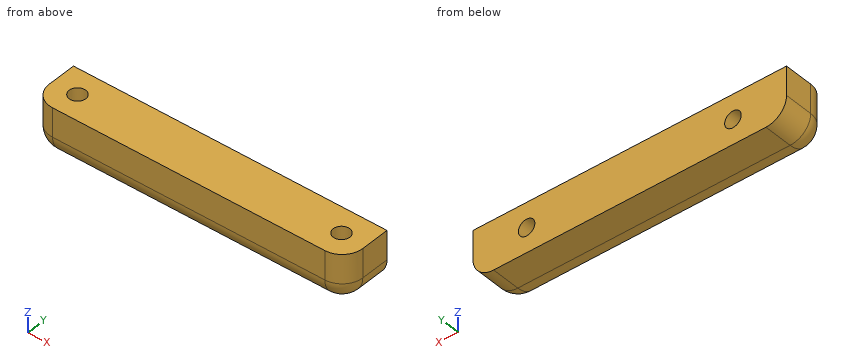
```python
from build123d import *

# Parameters (mm, degrees)
SKETCH1_W           = 76
SKETCH1_H           = 12
BOSS_EXTRUDE1_DEPTH = 6
SKETCH2_R           = 2
CUT_EXTRUDE1_DEPTH  = 8.5
SKETCH3_R           = 2
CUT_EXTRUDE2_DEPTH  = 8.5
FILLET1_R           = 5


with BuildPart() as part:
    # Sketch1 → Boss-Extrude1 (new, symmetric)
    with BuildSketch(Plane.XY):
        Rectangle(SKETCH1_W, SKETCH1_H)
    extrude(amount=BOSS_EXTRUDE1_DEPTH, both=True)

    # Sketch2 → Cut-Extrude1 (cut)
    with BuildSketch(Plane.XY.offset(6)):
        with Locations((-32, 0)):
            Circle(SKETCH2_R)
        with Locations((32, 0)):
            Circle(SKETCH2_R)
    extrude(amount=-CUT_EXTRUDE1_DEPTH, mode=Mode.SUBTRACT)

    # Sketch3 → Cut-Extrude2 (cut)
    with BuildSketch(Plane(origin=(0, 6, 0), x_dir=(1, 0, 0), z_dir=(0, 1, 0))):
        with Locations(Location((-25, 0, 0), (0, 0, 270))):
            Circle(SKETCH3_R)
        with Locations(Location((25, 0, 0), (0, 0, 270))):
            Circle(SKETCH3_R)
    extrude(amount=-CUT_EXTRUDE2_DEPTH, mode=Mode.SUBTRACT)

    # Fillet1
    fillet1_edges = [part.edges().sort_by_distance(p)[0] for p in [
        (38, 0, -6),
        (0, -6, -6),
        (-38, 0, -6),
        (38, -6, 0),
        (-38, -6, 0),
    ]]
    fillet(fillet1_edges, radius=FILLET1_R)


solid = part.part
```
Model file for the job. Use its own axes, mm. Coordinates: 2 decimals unless noted, no trailing zeros. Order: outer loops, then holes, each group sorted by start corner. A loop starts at its lowest first (then second) coordinate and runs counter-clockwise, first axis right, second up. Notation, with made-up numbers: (-7, -33.75) - (9, -33.75) arc R12 ccw to (9, -11.75) - close; hole circle Ø3 at (-1, 75.25). An arc over 180 degrees is marked (long way). Return JSON: item names as keys, results as strings. Group by question number.
1) Saw through at B-B, the plane z = 0. Write the cut outline in (x, y), plus the area to 3 significant figures.
2) Saw through at D-D, the plane y = 2.75. Write the cut outline in (x, z), plus the area to 3 significant figures.
3) Saw through at C-C, the plane x = 32. Write the cut outline in (y, z), plus the area to 3 significant figures.
4) Flat gauge pins, fed straight in: P1, Ø3, axis at y = -2.5, z = -2.5, coming from the -X side; P2, Ø3, axis at x = 25, z = 0, coming from the +Y side. Where does each tip first touch, or does it go through?
5) Probe line 1 (X direction, y = 3, z = 0); line 2 (X direction, y = 4.5, z = -1.5); line 3 (X direction, y = -0.75, z = -0.25). List the from-to ranges inside material, lowest first. Write a range as from..to.
6) Saw through at A-A, the plane y = 0. Write the cut outline in (x, z).
Values found:
{
 "1": {"outline": "(-38, -1) arc R5 ccw to (-33, -6) - (33, -6) arc R5 ccw to (38, -1) - (38, 6) - (27, 6) - (27, -2.5) - (23, -2.5) - (23, 6) - (-23, 6) - (-23, -2.5) - (-27, -2.5) - (-27, 6) - (-38, 6) - close; hole circle Ø4 at (-32, 0); hole circle Ø4 at (32, 0)", "area": "808 mm²"},
 "2": {"outline": "(-38, -1) arc R5 ccw to (-33, -6) - (33, -6) arc R5 ccw to (38, -1) - (38, 6) - (-38, 6) - close; hole circle Ø4 at (-25, 0); hole circle Ø4 at (25, 0)", "area": "876 mm²"},
 "3": {"outline": "(-6, -1) arc R5 ccw to (-1, -6) - (6, -6) - (6, 6) - (2, 6) - (2, -2.5) - (-2, -2.5) - (-2, 6) - (-6, 6) - close", "area": "105 mm²"},
 "4": {"P1": "stops at x = -37.96", "P2": "stops at y = -2.5"},
 "5": {"line 1": "x = -38..-27, -23..23, 27..38", "line 2": "x = -37.97..-26.32, -23.68..23.68, 26.32..37.97", "line 3": "x = -38..-33.85, -30.15..-26.98, -23.02..23.02, 26.98..30.15, 33.85..38"},
 "6": {"outline": "(-38, -1) arc R5 ccw to (-33, -6) - (33, -6) arc R5 ccw to (38, -1) - (38, 6) - (34, 6) - (34, -2.5) - (30, -2.5) - (30, 6) - (-30, 6) - (-30, -2.5) - (-34, -2.5) - (-34, 6) - (-38, 6) - close; hole circle Ø4 at (-25, 0); hole circle Ø4 at (25, 0)"}
}
